from build123d import *

# Parameters (mm, degrees)
F0_W     = 75
F0_H     = 15
F0_R     = 4.05
F0_R_2   = 1.75
F0_R_3   = 4.5
F1_DEPTH = 8
F0_H_2   = 3
F2_DEPTH = 23
F3_R     = 1.75
F4_DEPTH = 25


with BuildPart() as f1:
    # F0 (on Top) → F1 (new body)
    with BuildSketch(Plane.XY):
        Rectangle(F0_W, F0_H)
        with Locations((-25, 0)):
            Circle(F0_R, mode=Mode.SUBTRACT)
        with Locations((-12.5, 0)):
            Circle(F0_R_2, mode=Mode.SUBTRACT)
        Circle(F0_R_3, mode=Mode.SUBTRACT)
        with Locations((12.5, 0)):
            Circle(F0_R_2, mode=Mode.SUBTRACT)
        with Locations((25, 0)):
            Circle(F0_R, mode=Mode.SUBTRACT)
    extrude(amount=F1_DEPTH)

    # F0 (on Top) → F2 (join)
    with BuildSketch(Plane.XY):
        with Locations((0, 9)):
            Rectangle(F0_W, F0_H_2)
        with Locations((0, -9)):
            Rectangle(F0_W, F0_H_2)
    extrude(amount=F2_DEPTH)

    # F3 (on face) → F4 (cut)
    with BuildSketch(Plane.XZ.offset(10.5)):
        with Locations((-28.125, 15.5)):
            Circle(F3_R)
        with Locations((0, 15.5)):
            Circle(F3_R)
        with Locations((28.125, 15.5)):
            Circle(F3_R)
    extrude(amount=-F4_DEPTH, mode=Mode.SUBTRACT)


solid = f1.part
Can you work these out from the model? Positions are in its coordinate system, mm. A direction names the side the tool comes from. Coordinates: 2 decimals unless noted, no trailing zeros. Write each loop counter-clockwise with the first axis right and the second up, starting at its lowest first coordinate (ties: lowest second). Pieces come first, ordered by that corner, then holes. Notation, with made-up numbers: (18, -30.75) - (75, -30.75) arc R22 ccw to (75, -9.75) - close; hole circle Ø8 at (35, 13). An arc over 180 degrees is marked (long way). Return JSON: item names as keys, results as strings. Group by question number.
Item 1: If we section it at B-B (z = 7.25): Write out the boundary of the cut face in (x, y).
Item 2: Which directions (+Z, -Z, +X, -X, +Y, -Y) give clear straight access to the entire face, cutting with the end or side of a thin tool? Please do faces 5 (the face through (-1, 10.5, 11)), 6 (the face through (-1, -7.5, 12)).
Item 3: If we section it at D-D (z = 15.5): Count the separate pieces of the cut face and the enclosed holes in it, then the cut area to 3 significant figures.
Item 4: If we section it at A-A (x = 12.5): Write out the boundary of the cut face in (y, z).
Item 5: If we section it at C-C (y = 0): Write out the boundary of the cut face in (x, z).
Item 6: I'm going to push flat-ended pins straight in: pin 1 Ø6.5 at (x, y) = (-25, 0) entering from -Z; pin 2 Ø4.5 at (x, y) = (11, 3) entering from +Z. Where does each tip first touch, or does it pass through?
Item 7: Please list where these lines run through material, in increasing order: probe 1 along Y at (x, z) = (-12.5, 2); probe 2 along Y at (x, z) = (-9, 16.25); probe 3 along X at (y, z) = (-3, 2).
Item 8: We'd pull the mould along Y, two halves only. Please class faces 1 (the face through (-29.4, 9, 16.7)), 2 (the face through (28.86, 1.22, 3.94)), 3 (the face through (-1, -10.5, 11)), 4 (the face through (-1, 5, 8)): pulls with the +Y half, pulls with the -Y half, needs draft (parallel to the pull), parting line crosses it, or undercut.
Return value:
{
 "1": {"outline": "(-37.5, -10.5) - (37.5, -10.5) - (37.5, 10.5) - (-37.5, 10.5) - close; hole circle Ø8.1 at (-25, 0); hole circle Ø3.5 at (-12.5, 0); hole circle Ø9 at (0, 0); hole circle Ø3.5 at (12.5, 0); hole circle Ø8.1 at (25, 0)"},
 "2": {"face 5": "+Z, -Z, +X, -X, +Y", "face 6": "+Z, +X, -X"},
 "3": {"separate pieces": "8", "enclosed holes": "0", "area": "387 mm^2"},
 "4": {"outline": "(-10.5, 0) - (-1.75, 0) - (-1.75, 8) - (-7.5, 8) - (-7.5, 23) - (-10.5, 23) - close; (1.75, 0) - (10.5, 0) - (10.5, 23) - (7.5, 23) - (7.5, 8) - (1.75, 8) - close"},
 "5": {"outline": "(-37.5, 0) - (-29.05, 0) - (-29.05, 8) - (-37.5, 8) - close; (-20.95, 0) - (-14.25, 0) - (-14.25, 8) - (-20.95, 8) - close; (-10.75, 0) - (-4.5, 0) - (-4.5, 8) - (-10.75, 8) - close; (4.5, 0) - (10.75, 0) - (10.75, 8) - (4.5, 8) - close; (14.25, 0) - (20.95, 0) - (20.95, 8) - (14.25, 8) - close; (29.05, 0) - (37.5, 0) - (37.5, 8) - (29.05, 8) - close"},
 "6": {"pin 1": "passes through", "pin 2": "stops at z = 8"},
 "7": {"probe 1": "y = -10.5 to -1.75, 1.75 to 10.5", "probe 2": "y = -10.5 to -7.5, 7.5 to 10.5", "probe 3": "x = -37.5 to -27.72, -22.28 to -3.35, 3.35 to 22.28, 27.72 to 37.5"},
 "8": {"face 1": "needs draft", "face 2": "undercut", "face 3": "pulls with the -Y half", "face 4": "undercut"}
}
